The figure shows three views and two pictorial views of one solid part (mm, origin at its lowest corner). Answer the questions. Coordinates: 2 decimals unless noted, no trailing zeros. Loops run counter-clockwise (first coordinate to the right, second up) from the corner with the lowest first, then second, coordinate; pieces in that order, holes last. Notation, with made-up numbers: M -21,-16 L -12,-16 A16 cw -12,-3 Z; hole C 49.5,57 d1. An arc over 180 degrees is marked long. Return JSON: item names as keys, results as strings. Group by question number.
1. Section B-B (x = 15) is taken. Write down the section's boundary in (y, z).
2. Section C-C (x = 6.75) is taken. Write down the section's boundary in (y, z).
3. Straight lines are drawn through the part: L1, parallel to Y at x = 15, z = 1; L2, parallel to Y at x = 14, z = 2.1; L3, parallel to X at y = 4, z = 2.45. For each, find the intervals that lie inside material, in ascending order. Write a range as from..to.
4. Section D-D (y = 35.5) is taken. Write down the section's boundary in (x, z), then the cut area to 3 significant figures.
5. Section A-A (z = 2.5) is taken. Write down the section's boundary in (x, y), then the cut area to 3 significant figures.
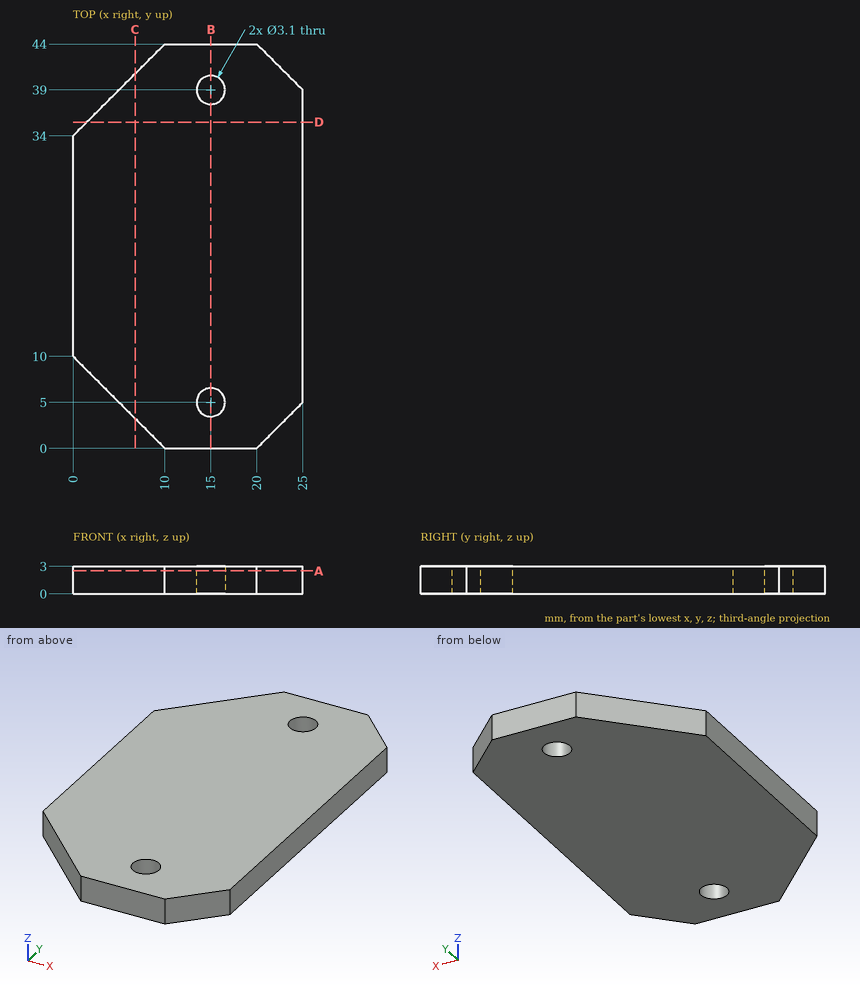
Worked out:
{
 "1": {"outline": "M 0,0 L 3.45,0 L 3.45,3 L 0,3 Z; M 6.55,0 L 37.45,0 L 37.45,3 L 6.55,3 Z; M 40.55,0 L 44,0 L 44,3 L 40.55,3 Z"},
 "2": {"outline": "M 3.25,0 L 40.75,0 L 40.75,3 L 3.25,3 Z"},
 "3": {"L1": "0..3.45, 6.55..37.45, 40.55..44", "L2": "0..3.82, 6.18..37.82, 40.18..44", "L3": "6..13.82, 16.18..24"},
 "4": {"outline": "M 1.5,0 L 25,0 L 25,3 L 1.5,3 Z", "area": "70.5 mm^2"},
 "5": {"outline": "M 0,10 L 10,0 L 20,0 L 25,5 L 25,39 L 20,44 L 10,44 L 0,34 Z; hole C 15,5 d3.1; hole C 15,39 d3.1", "area": "960 mm^2"}
}
